Part print with two shaded views. Sizes in mm from the minimum x, y, z corner. A direction names the side the tool comes from. Round coordinates to 2 decimals unless told otherwise and drop trailing zeros. Order: outer loops, then holes, each group sorted by start corner. A loop starts at its lowest first (then second) coordinate and runs counter-clockwise, first axis right, second up. Notation, with made-up numbers: M -8.75,-20 L 47.25,-20 A22 cw 47.25,-10 Z; hole C 20,-3 d8. An arc over 180 degrees is marked long. Put each result on its own line as item: value.
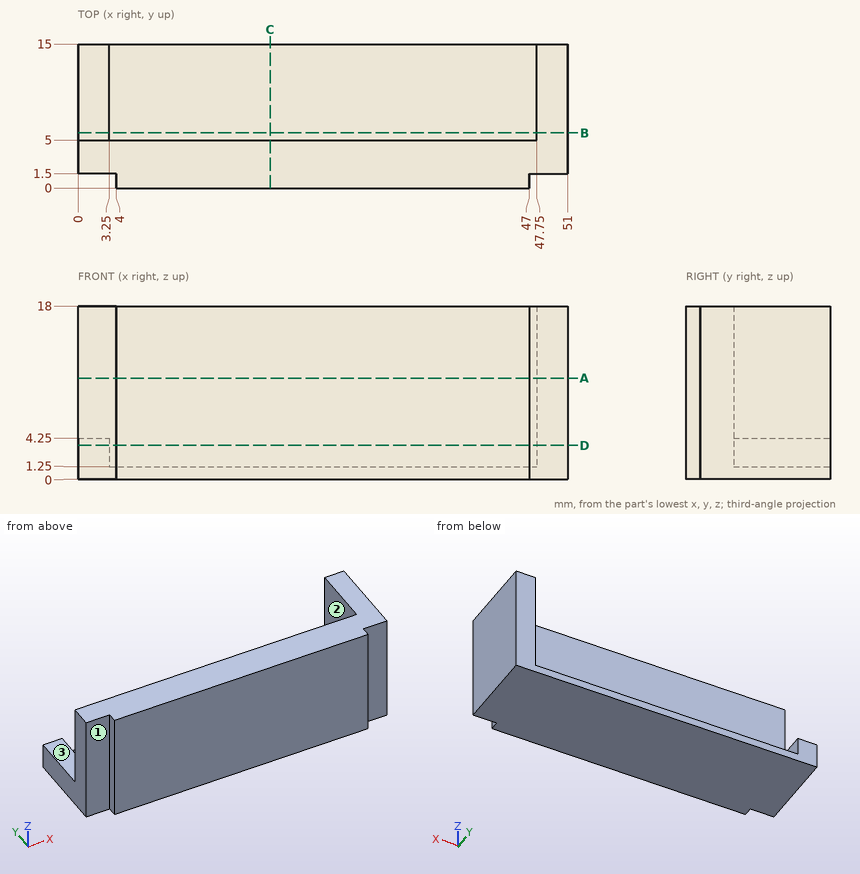
Item 1: Pin check, flat tips, straight feed: P1, Ø1.6, axis at x = 1, y = 8, coming from the +Z side; P2, Ø2, axis at x = 23.5, z = 16, coming from the +Y side; P3, Ø1.6, axis at y = 0.5, z = 8.5, coming from the -X side. Stop position of each tip, or through.
Answers below:
P1: z = 4.25
P2: y = 5
P3: x = 4
Item 2: Band-saw the part on B-B on y = 5.75. Give the cut face in (x, z), and give its area (3 significant figures).
Answers below:
outline: M 0,0 L 51,0 L 51,18 L 47.75,18 L 47.75,1.25 L 3.25,1.25 L 3.25,4.25 L 0,4.25 Z
area: 128 mm²
Item 3: Band-saw the part on A-A on z = 10.5. Give the cut face in (x, y).
Answers below:
outline: M 0,1.5 L 4,1.5 L 4,0 L 47,0 L 47,1.5 L 51,1.5 L 51,15 L 47.75,15 L 47.75,5 L 0,5 Z
Item 4: Probe line 1 along Y through (x, z) = (12, 8.5); line 2 along X through (y, z) = (13, 9.75); line 3 along Z through (x, y) = (3, 6.5). List the from-to ranges inside material, lowest first. Write a range as [from, to].
Answers below:
line 1: [0, 5]
line 2: [47.75, 51]
line 3: [0, 4.25]
Item 5: Band-saw the part on C-C on x = 20. Give the cut face in (y, z).
Answers below:
outline: M 0,0 L 15,0 L 15,1.25 L 5,1.25 L 5,18 L 0,18 Z
Item 6: Band-saw the part on D-D on z = 3.5. Give the cut face in (x, y).
Answers below:
outline: M 0,1.5 L 4,1.5 L 4,0 L 47,0 L 47,1.5 L 51,1.5 L 51,15 L 47.75,15 L 47.75,5 L 3.25,5 L 3.25,15 L 0,15 Z
Item 7: Tool access for the marked faces 1, 2 and 3: list every direction of +Z, -Z, +X, -X, +Y, -Y with a clear straight run to the whole face (end or side of a thin tool).
Answers below:
face 1: +Z, -Z, -X, -Y
face 2: +Z, +Y
face 3: +Z, -X, +Y
